from build123d import *

# Parameters (mm, degrees)
SKETCH1_W           = 30
SKETCH1_H           = 17.5
BOSS_EXTRUDE1_DEPTH = 4
SKETCH2_W           = 30
SKETCH2_H           = 6
BOSS_EXTRUDE2_DEPTH = 1.601
SKETCH3_W           = 10
SKETCH3_H           = 3
BOSS_EXTRUDE3_DEPTH = 18.7
SKETCH4_W           = 10
SKETCH4_H           = 3
BOSS_EXTRUDE4_DEPTH = 17.099
SKETCH5_W           = 10
SKETCH5_H           = 3
BOSS_EXTRUDE5_DEPTH = 1.601
FILLET1_R           = 2
CUT_EXTRUDE1_REACH  = 42.318
SKETCH6_R           = 1.4224
CUT_EXTRUDE2_REACH  = 42.318
SKETCH7_R           = 1.4224
SKETCH9_W           = 10
SKETCH9_H           = 3
SKETCH9_W_2         = 9.9
SKETCH9_H_2         = 2.9
CUT_EXTRUDE3_DEPTH  = 17.099


with BuildPart() as part:
    # Sketch1 → Boss-Extrude1 (new body)
    with BuildSketch(Plane(origin=(0, 0, 0), x_dir=(1, 0, 0), z_dir=(0, 1, 0))):
        with Locations((15, 8.75)):
            Rectangle(SKETCH1_W, SKETCH1_H)
    extrude(amount=BOSS_EXTRUDE1_DEPTH)

    # Sketch2 → Boss-Extrude2 (add)
    with BuildSketch(Plane(origin=(0, 4, 0), x_dir=(1, 0, 0), z_dir=(0, 1, 0))):
        with Locations((15, 14.5)):
            Rectangle(SKETCH2_W, SKETCH2_H)
    extrude(amount=BOSS_EXTRUDE2_DEPTH)

    # Sketch3 → Boss-Extrude3 (add)
    with BuildSketch(Plane(origin=(0, 4, 0), x_dir=(1, 0, 0), z_dir=(0, 1, 0))):
        with Locations((5, 1.5)):
            Rectangle(SKETCH3_W, SKETCH3_H)
        with Locations((25, 1.5)):
            Rectangle(SKETCH3_W, SKETCH3_H)
    extrude(amount=BOSS_EXTRUDE3_DEPTH)

    # Sketch4 → Boss-Extrude4 (add)
    with BuildSketch(Plane(origin=(0, 5.601, 0), x_dir=(1, 0, 0), z_dir=(0, 1, 0))):
        with Locations((5, 16)):
            Rectangle(SKETCH4_W, SKETCH4_H)
        with Locations((25, 16)):
            Rectangle(SKETCH4_W, SKETCH4_H)
    extrude(amount=BOSS_EXTRUDE4_DEPTH)

    # Sketch5 → Boss-Extrude5 (add)
    with BuildSketch(Plane(origin=(0, 4, 0), x_dir=(1, 0, 0), z_dir=(0, 1, 0))):
        with Locations((15, 1.5)):
            Rectangle(SKETCH5_W, SKETCH5_H)
    extrude(amount=BOSS_EXTRUDE5_DEPTH)

    # Fillet1
    fillet1_edges = [part.edges().sort_by_distance(p)[0] for p in [
        (15, 0, -17.5),
        (30, 0, -8.75),
        (15, 0, 0),
        (10, 14.1505, -17.5),
        (5, 22.7, -17.5),
        (0, 0, -8.75),
        (15, 5.601, -17.5),
        (20, 14.1505, -17.5),
        (25, 22.7, -17.5),
        (0, 11.35, -17.5),
        (30, 11.35, -17.5),
    ]]
    fillet(fillet1_edges, radius=FILLET1_R)

    # Sketch6 → Cut-Extrude1 (cut, up to next)
    with BuildSketch(Plane.XY.offset(-14.5), mode=Mode.PRIVATE) as cut_extrude1_sk1:
        with Locations((5, 19.2)):
            Circle(SKETCH6_R)
    cut_extrude1_tool1 = extrude(cut_extrude1_sk1.sketch, amount=-CUT_EXTRUDE1_REACH, mode=Mode.PRIVATE) & part.part
    # Sketch6 → Cut-Extrude1 (cut, up to next)
    with BuildSketch(Plane.XY.offset(-14.5), mode=Mode.PRIVATE) as cut_extrude1_sk2:
        with Locations((25, 19.2)):
            Circle(SKETCH6_R)
    cut_extrude1_tool2 = extrude(cut_extrude1_sk2.sketch, amount=-CUT_EXTRUDE1_REACH, mode=Mode.PRIVATE) & part.part
    # Sketch6 → Cut-Extrude1 (cut, up to next)
    with BuildSketch(Plane.XY.offset(-14.5), mode=Mode.PRIVATE) as cut_extrude1_sk3:
        with Locations((5, 14.2)):
            Circle(SKETCH6_R)
    cut_extrude1_tool3 = extrude(cut_extrude1_sk3.sketch, amount=-CUT_EXTRUDE1_REACH, mode=Mode.PRIVATE) & part.part
    # Sketch6 → Cut-Extrude1 (cut, up to next)
    with BuildSketch(Plane.XY.offset(-14.5), mode=Mode.PRIVATE) as cut_extrude1_sk4:
        with Locations((25, 14.2)):
            Circle(SKETCH6_R)
    cut_extrude1_tool4 = extrude(cut_extrude1_sk4.sketch, amount=-CUT_EXTRUDE1_REACH, mode=Mode.PRIVATE) & part.part
    add(cut_extrude1_tool1.solids().sort_by_distance((5, 19.2, -14.5))[0], mode=Mode.SUBTRACT)
    add(cut_extrude1_tool2.solids().sort_by_distance((25, 19.2, -14.5))[0], mode=Mode.SUBTRACT)
    add(cut_extrude1_tool3.solids().sort_by_distance((5, 14.2, -14.5))[0], mode=Mode.SUBTRACT)
    add(cut_extrude1_tool4.solids().sort_by_distance((25, 14.2, -14.5))[0], mode=Mode.SUBTRACT)

    # Sketch7 → Cut-Extrude2 (cut, up to next)
    with BuildSketch(Plane(origin=(0, 0, -3), x_dir=(-1, 0, 0), z_dir=(0, 0, -1)), mode=Mode.PRIVATE) as cut_extrude2_sk1:
        with Locations(Location((-5, 19.2, 0), (0, 0, 180))):
            Circle(SKETCH7_R)
    cut_extrude2_tool1 = extrude(cut_extrude2_sk1.sketch, amount=-CUT_EXTRUDE2_REACH, mode=Mode.PRIVATE) & part.part
    # Sketch7 → Cut-Extrude2 (cut, up to next)
    with BuildSketch(Plane(origin=(0, 0, -3), x_dir=(-1, 0, 0), z_dir=(0, 0, -1)), mode=Mode.PRIVATE) as cut_extrude2_sk2:
        with Locations((-25.150725931, 19.2)):
            Circle(SKETCH7_R)
    cut_extrude2_tool2 = extrude(cut_extrude2_sk2.sketch, amount=-CUT_EXTRUDE2_REACH, mode=Mode.PRIVATE) & part.part
    # Sketch7 → Cut-Extrude2 (cut, up to next)
    with BuildSketch(Plane(origin=(0, 0, -3), x_dir=(-1, 0, 0), z_dir=(0, 0, -1)), mode=Mode.PRIVATE) as cut_extrude2_sk3:
        with Locations((-25.150725931, 14.2)):
            Circle(SKETCH7_R)
    cut_extrude2_tool3 = extrude(cut_extrude2_sk3.sketch, amount=-CUT_EXTRUDE2_REACH, mode=Mode.PRIVATE) & part.part
    # Sketch7 → Cut-Extrude2 (cut, up to next)
    with BuildSketch(Plane(origin=(0, 0, -3), x_dir=(-1, 0, 0), z_dir=(0, 0, -1)), mode=Mode.PRIVATE) as cut_extrude2_sk4:
        with Locations(Location((-5, 14.2, 0), (0, 0, 180))):
            Circle(SKETCH7_R)
    cut_extrude2_tool4 = extrude(cut_extrude2_sk4.sketch, amount=-CUT_EXTRUDE2_REACH, mode=Mode.PRIVATE) & part.part
    add(cut_extrude2_tool1.solids().sort_by_distance((5, 19.2, -3))[0], mode=Mode.SUBTRACT)
    add(cut_extrude2_tool2.solids().sort_by_distance((25.150726, 19.2, -3))[0], mode=Mode.SUBTRACT)
    add(cut_extrude2_tool3.solids().sort_by_distance((25.150726, 14.2, -3))[0], mode=Mode.SUBTRACT)
    add(cut_extrude2_tool4.solids().sort_by_distance((5, 14.2, -3))[0], mode=Mode.SUBTRACT)

    # Sketch9 → Cut-Extrude3 (cut)
    # profile 1 of 2: a face of its own
    with BuildSketch(Plane(origin=(0, 22.7, 0), x_dir=(1, 0, 0), z_dir=(0, 1, 0))):
        with Locations((25, 1.5)):
            Rectangle(SKETCH9_W, SKETCH9_H)
        with Locations((25, 1.5)):
            Rectangle(SKETCH9_W_2, SKETCH9_H_2, mode=Mode.SUBTRACT)
    # profile 2 of 2: a face of its own
    with BuildSketch(Plane(origin=(0, 22.7, 0), x_dir=(1, 0, 0), z_dir=(0, 1, 0))):
        with Locations((5, 1.5)):
            Rectangle(SKETCH9_W, SKETCH9_H)
        with Locations((5, 1.5)):
            Rectangle(SKETCH9_W_2, SKETCH9_H_2, mode=Mode.SUBTRACT)
    extrude(amount=-CUT_EXTRUDE3_DEPTH, mode=Mode.SUBTRACT)


solid = part.part
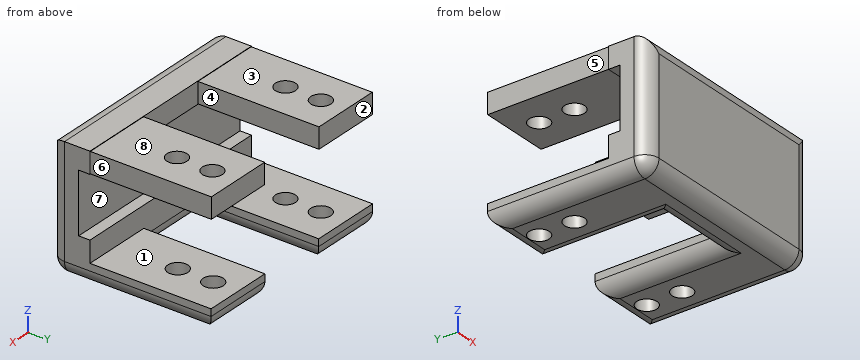
Input: part model. Units: mm. Frame: model coordinates. Face numbers are marked on the shaded views. A direction names the side the tool comes from. Coordinates: 2 decimals unless noted, no trailing zeros. Loops run counter-clockwise (first coordinate to the right, second up) from the corner with the lowest first, then second, coordinate; pieces in that order, holes last. Notation, with made-up numbers: (-37, -19.75) -> (11, -19.75) arc R23 cw to (11, -0.75) -> close; hole circle Ø9 at (32, 67). An arc over 180 degrees is marked (long way). One line per item, written item: value.
(1) Ray query, line 1 along Y through (x, z) = (5, -15.15); line 2 along Z through (x, y) = (23.75, 11.5); line 3 along Y through (x, z) = (25, -16.15). Return the intervals inside material, ascending.
Answer below:
line 1: y = 0 to 12.78, 15.62 to 17.78, 20.62 to 22.7
line 2: z = -17.5 to -14.5, -2.95 to -0.05
line 3: y = 0.11 to 12.78, 15.62 to 17.78, 20.62 to 22.59
(2) Cut plane C-C (x = 17.5). Output: boundary loops of the cut face in (y, z), then the cut area to 3 significant figures.
Answer below:
outline: (0, -15.5) arc R2 ccw to (2, -17.5) -> (3.6, -17.5) arc R2 ccw to (5.6, -15.5) -> (5.6, -11.5) -> (4, -11.5) -> (4, -3) -> (5.6, -3) -> (5.6, 0) -> (2, 0) arc R2 ccw to (0, -2) -> close
area: 81.8 mm2
(3) Cut plane A-A (x = 5). Give the number of separate pieces and of enclosed holes in the cut face, then the cut area to 3 significant figures.
Answer below:
separate pieces: 5
enclosed holes: 0
area: 149 mm2
(4) Set-up query: the marked faces 4, 5, 6, 7 and 8. Return all of +Z, -Z, +X, -X, +Y, -Y with unobstructed straight access to the full face (end or side cutting, diameter ignored); none if empty.
Answer below:
face 4: +Z, +Y
face 5: +Z, -X, +Y
face 6: +Z, +X, +Y
face 7: +X, -X, +Y
face 8: +Z, +X, -X, +Y
(5) Cut plane B-B (y = 10.75). Output: boundary loops of the cut face in (x, z).
Answer below:
outline: (0, -15.5) arc R2 ccw to (2, -17.5) -> (8, -17.5) arc R2 ccw to (10, -15.5) -> (10, -14.5) -> (0, -14.5) -> close; (0.05, -2.95) -> (9.95, -2.95) -> (9.95, -0.05) -> (0.05, -0.05) -> close; (20, -15.5) arc R2 ccw to (22, -17.5) -> (28, -17.5) arc R2 ccw to (30, -15.5) -> (30, -14.5) -> (20, -14.5) -> close; (20.05, -2.95) -> (29.95, -2.95) -> (29.95, -0.05) -> (20.05, -0.05) -> close
(6) Draft query along Z for the marked faces 1, 2 and 3. Return one class per face: pulls with the +Z half, pulls with the -Z half, needs draft (parallel to the pull), parting line crosses it, or undercut.
Answer below:
face 1: undercut
face 2: needs draft
face 3: pulls with the +Z half
(7) Pin query (flat end, axial travel): pin 1 Ø1.3 at (x, y) = (19.5, 5) entering from -Z; pin 2 Ø10 at (x, z) = (19.5, -6.5) entering from +Y; pin 3 Ø2.5 at (x, y) = (5, 19.2) entering from +Z; pin 4 Ø1.5 at (x, z) = (21, -6.5) entering from +Y. Return the tip coordinate at first contact, or that it passes through.
Answer below:
pin 1: stops at z = -17.35
pin 2: stops at y = 22.7
pin 3: passes through
pin 4: stops at y = 4
